Autodesk Inventor part; units mm, degrees
ref_plane "Work Plane1" through (0, 0, 38.1) normal (0, 0, 1) x (1, 0, 0)
ref_plane "YZ Plane" through (0, 0, 0) normal (1, 0, 0) x (0, 1, 0)
ref_plane "XZ Plane" through (0, 0, 0) normal (0, 1, 0) x (-1, 0, 0)
sketch "Sketch1" plane through (0, 0, 0) normal (0, 0, 1) x (1, 0, 0)
  circle A0 centre (0, 0) radius 14.2875
  circle A1 centre (0, 0) radius 17.4625
  circle A2 centre (0, 0) radius 19.05
  circle A3 centre (0, 0) radius 22.8953
  circle A4 centre (0, 0) radius 24.4828
  circle A5 centre (0, 0) radius 27.6578
  circle A6 centre (0, 0) radius 29.2453
  dimension "d0" = 28.575
  dimension "d1" = 34.925
  dimension "d2" = 38.1
  dimension "d3" = 45.7905
  dimension "d4" = 48.9655
  dimension "d5" = 55.3155
  dimension "d6" = 58.4905
extrude "Extrusion1" add sketch "Sketch1" along normal blind 38.1 contours A0 | A1 | A2 | A3 | A4 | A5 | A6
sketch "Sketch2" plane through (0, 0, 0) normal (0, 1, 0) x (-1, 0, 0)
  circle A0 centre (0, 19.05) radius 14.2875
  line L0 (29.2453, 0) -> (-29.2453, 0)
  point P0 (0, 0)
  dimension "d9" = 19.05
  dimension "d10" = 28.575
extrude "Extrusion2" add sketch "Sketch2" along normal blind 50.8
shell "Shell1" thickness 1.5875 removed faces 3 at (13.4185, 9.6773, 0) at (13.4185, 9.6773, 38.1) at (-3.9719, 50.8, 19.2449)
sketch "Sketch3" plane through (0, 0, 0) normal (0, 0, 1) x (1, 0, 0)
  circle A0 centre (0, 0) radius 14.2875
  circle A1 centre (0, 0) radius 17.4625
  circle A2 centre (0, 0) radius 19.05
  circle A3 centre (0, 0) radius 22.8953
  circle A4 centre (0, 0) radius 24.4828
  circle A5 centre (0, 0) radius 27.6578
  circle A6 centre (0, 0) radius 29.2453
  dimension "d14" = 28.575
  dimension "d15" = 34.925
  dimension "d16" = 38.1
  dimension "d17" = 45.7905
  dimension "d18" = 48.9655
  dimension "d19" = 55.3155
  dimension "d20" = 58.4905
extrude "Extrusion3" add sketch "Sketch3" along normal blind 1.5875 contours A5
ref_plane "Work Plane1" through (0, 0, 38.1) normal (0, 0, 1) x (1, 0, 0)
sketch "Sketch4" plane through (0, 0, 38.1) normal (0, 0, 1) x (1, 0, 0)
  circle A0 centre (0, 0) radius 14.2875
  circle A1 centre (0, 0) radius 17.4625
  circle A2 centre (0, 0) radius 19.05
  circle A3 centre (0, 0) radius 22.8953
  circle A4 centre (0, 0) radius 24.4828
  circle A5 centre (0, 0) radius 27.6578
  circle A6 centre (0, 0) radius 29.2453
  dimension "d24" = 28.575
  dimension "d25" = 34.925
  dimension "d26" = 38.1
  dimension "d27" = 45.7905
  dimension "d28" = 48.9655
  dimension "d29" = 55.3155
  dimension "d30" = 58.4905
extrude "Extrusion4" add sketch "Sketch4" against normal blind 1.5875 contours A5
properties part number "Exhaust" material "Stainless Steel"
Part model, mm, in its own coordinate system. A direction names the side the tool comes from. Round coordinates to 2 decimals unless told otherwise and drop trailing zeros. Order: outer loops, then holes, each group sorted by start corner. A loop starts at its lowest first (then second) coordinate and runs counter-clockwise, first axis right, second up. Notation, with made-up numbers: (-29, 2.25) -> (12, 2.25) arc R23 cw to (12, 22.25) -> close; hole circle Ø1 at (-32.5, 3). An arc over 180 degrees is marked (long way). Put each result on its own line as item: value.
Q1. Pin check, flat tips, straight feed: pin 1 Ø8 at (y, z) = (27, 26) entering from -X; pin 2 Ø1.5 at (y, z) = (28, 16.5) entering from +X; pin 3 Ø3 at (y, z) = (2.5, 4.5) entering from -X. Stop position of each tip, or through.
From the geometry:
pin 1: stops at x = -18.06
pin 2: stops at x = 14.17
pin 3: stops at x = -29.23
Q2. Band-saw the part on A-A (x = 0). Give the cut face in (y, z), and give its area (3 significant figures).
From the geometry:
outline: (-29.25, 0) -> (-24.48, 0) -> (-24.48, 1.59) -> (-27.66, 1.59) -> (-27.66, 36.51) -> (-24.48, 36.51) -> (-24.48, 38.1) -> (-29.25, 38.1) -> close; (24.48, 0) -> (29.25, 0) -> (29.25, 4.76) -> (50.8, 4.76) -> (50.8, 6.35) -> (27.66, 6.35) -> (27.66, 1.59) -> (24.48, 1.59) -> close; (24.48, 36.51) -> (27.66, 36.51) -> (27.66, 31.75) -> (50.8, 31.75) -> (50.8, 33.34) -> (29.25, 33.34) -> (29.25, 38.1) -> (24.48, 38.1) -> close
area: 169 mm2
Q3. Wall check: line 1 (X direction, y = 43.5, z = 19.05); line 2 (Y direction, x = 0, z = 0.7); line 3 (Z direction, x = 26, y = 2.5). Give the ranges that are in metal, low to high. Write a range as [from, to].
From the geometry:
line 1: x = [-14.29, -12.7], [12.7, 14.29]
line 2: y = [-29.25, -24.48], [24.48, 29.25]
line 3: z = [0, 1.59], [36.51, 38.1]
Q4. Band-saw the part on C-C (z = 19.05). Give the cut face in (x, y).
From the geometry:
outline: (-14.29, 25.52) arc R29.25 ccw (long way) to (14.29, 25.52) -> (14.29, 50.8) -> (12.7, 50.8) -> (12.7, 24.57) arc R27.66 cw (long way) to (-12.7, 24.57) -> (-12.7, 50.8) -> (-14.29, 50.8) -> close
Q5. Tool access for faces 4 (the face through (23.352, 7.354, 37.317)), 5 (the face through (-5.86, 37.501, 30.317)), 6 (the face through (-10.4, -22.4, 36.512)): list every direction of +Z, -Z, +X, -X, +Y, -Y with a clear straight run to the whole face (end or side of a thin tool).
From the geometry:
face 4: +Z, -Z
face 5: +Y
face 6: none
Q6. Pull direction X, two halves, no side cores. Call faces 1 (the face through (-3.6, -27.422, 18.806)), 2 (the face through (-13.2, 37.98, 24.52)), 3 (the face through (-7, -24, 0)): pulls with the +X half, pulls with the -X half, needs draft (parallel to the pull), parting line crosses it, or undercut.
From the geometry:
face 1: undercut
face 2: parting line crosses it
face 3: needs draft
Q7. Band-saw the part on B-B (y = 0). Give the cut face in (x, z).
From the geometry:
outline: (-29.25, 0) -> (-24.48, 0) -> (-24.48, 1.59) -> (-27.66, 1.59) -> (-27.66, 36.51) -> (-24.48, 36.51) -> (-24.48, 38.1) -> (-29.25, 38.1) -> close; (24.48, 0) -> (29.25, 0) -> (29.25, 38.1) -> (24.48, 38.1) -> (24.48, 36.51) -> (27.66, 36.51) -> (27.66, 1.59) -> (24.48, 1.59) -> close
Q8. Band-saw the part on D-D (x = 18). Give the cut face in (y, z), and give its area (3 significant figures).
From the geometry:
outline: (-23.05, 0) -> (-16.6, 0) -> (-16.6, 1.59) -> (-21, 1.59) -> (-21, 36.51) -> (-16.6, 36.51) -> (-16.6, 38.1) -> (-23.05, 38.1) -> close; (16.6, 0) -> (23.05, 0) -> (23.05, 38.1) -> (16.6, 38.1) -> (16.6, 36.51) -> (21, 36.51) -> (21, 1.59) -> (16.6, 1.59) -> close
area: 184 mm2
